from build123d import *

# Parameters (mm, degrees)
F0_W     = 6.858
F0_H     = 2.54
F0_R     = 0.381
F0_W_2   = 0.762
F0_H_2   = 7.62
F1_DEPTH = 2.54


with BuildPart() as f1:
    # F0 (on Top) → F1 (new body)
    with BuildSketch(Plane.XY):
        with Locations((-12.065, 8.001)):
            Rectangle(F0_W, F0_H)
        with Locations((-12.065, -8.001)):
            Rectangle(F0_W, F0_H)
        Polygon((8.636, -13.97), (8.636, 13.97), (-8.636, 13.97), (-8.636, 9.271), (-8.636, 6.731), (-8.636, -6.731), (-8.636, -9.271), (-8.636, -13.97), align=None)
        with Locations((-6.98514, -12.7)):
            Circle(F0_R, mode=Mode.SUBTRACT)
        with Locations((-4.95312, -12.7)):
            Circle(F0_R, mode=Mode.SUBTRACT)
        with Locations((-6.95875, -6.35)):
            Rectangle(F0_W_2, F0_H_2, mode=Mode.SUBTRACT)
        with Locations((-4.9305, -6.35)):
            Rectangle(F0_W_2, F0_H_2, mode=Mode.SUBTRACT)
        with Locations((-2.9211, -12.7)):
            Circle(F0_R, mode=Mode.SUBTRACT)
        with Locations((-0.88908, -12.7)):
            Circle(F0_R, mode=Mode.SUBTRACT)
        with Locations((1.14294, -12.7)):
            Circle(F0_R, mode=Mode.SUBTRACT)
        with Locations((3.17496, -12.7)):
            Circle(F0_R, mode=Mode.SUBTRACT)
        with Locations((5.20698, -12.7)):
            Circle(F0_R, mode=Mode.SUBTRACT)
        with Locations((7.239, -12.7)):
            Circle(F0_R, mode=Mode.SUBTRACT)
        with Locations((-2.90225, -6.35)):
            Rectangle(F0_W_2, F0_H_2, mode=Mode.SUBTRACT)
        with Locations((-0.874, -6.35)):
            Rectangle(F0_W_2, F0_H_2, mode=Mode.SUBTRACT)
        with Locations((1.15425, -6.35)):
            Rectangle(F0_W_2, F0_H_2, mode=Mode.SUBTRACT)
        with Locations((3.1825, -6.35)):
            Rectangle(F0_W_2, F0_H_2, mode=Mode.SUBTRACT)
        with Locations((5.21075, -6.35)):
            Rectangle(F0_W_2, F0_H_2, mode=Mode.SUBTRACT)
        with Locations((7.239, -6.35)):
            Rectangle(F0_W_2, F0_H_2, mode=Mode.SUBTRACT)
        with Locations((-6.95875, 6.35)):
            Rectangle(F0_W_2, F0_H_2, mode=Mode.SUBTRACT)
        with Locations((-4.9305, 6.35)):
            Rectangle(F0_W_2, F0_H_2, mode=Mode.SUBTRACT)
        with Locations((-6.98514, 12.7)):
            Circle(F0_R, mode=Mode.SUBTRACT)
        with Locations((-4.95312, 12.7)):
            Circle(F0_R, mode=Mode.SUBTRACT)
        with Locations((-2.90225, 6.35)):
            Rectangle(F0_W_2, F0_H_2, mode=Mode.SUBTRACT)
        with Locations((-0.874, 6.35)):
            Rectangle(F0_W_2, F0_H_2, mode=Mode.SUBTRACT)
        with Locations((1.15425, 6.35)):
            Rectangle(F0_W_2, F0_H_2, mode=Mode.SUBTRACT)
        with Locations((3.1825, 6.35)):
            Rectangle(F0_W_2, F0_H_2, mode=Mode.SUBTRACT)
        with Locations((5.21075, 6.35)):
            Rectangle(F0_W_2, F0_H_2, mode=Mode.SUBTRACT)
        with Locations((7.239, 6.35)):
            Rectangle(F0_W_2, F0_H_2, mode=Mode.SUBTRACT)
        with Locations((-2.9211, 12.7)):
            Circle(F0_R, mode=Mode.SUBTRACT)
        with Locations((-0.88908, 12.7)):
            Circle(F0_R, mode=Mode.SUBTRACT)
        with Locations((1.14294, 12.7)):
            Circle(F0_R, mode=Mode.SUBTRACT)
        with Locations((3.17496, 12.7)):
            Circle(F0_R, mode=Mode.SUBTRACT)
        with Locations((5.20698, 12.7)):
            Circle(F0_R, mode=Mode.SUBTRACT)
        with Locations((7.239, 12.7)):
            Circle(F0_R, mode=Mode.SUBTRACT)
    extrude(amount=-F1_DEPTH)


solid = f1.part
Work out the finished part from the listing and answer in its coordinate system (mm). A direction names the side the tool comes from. Round coordinates to 2 decimals unless told otherwise and drop trailing zeros. Loops run counter-clockwise (first coordinate to the right, second up) from the corner with the lowest first, then second, coordinate; pieces in that order, holes last. Notation, with made-up numbers: (73.25, 0) -> (127.25, 0) arc R14 cw to (127.25, 16) -> close; hole circle Ø5 at (-5.75, 28). An arc over 180 degrees is marked (long way). Use one line per item in the form item = value.
(1) Straight lines are drawn through the part: line 1 (Y direction, x = -5, z = -0.6); line 2 (Y direction, x = 7, z = -1.15); line 3 (Y direction, x = -13, z = -1). For each, find the intervals that lie inside material, in ascending order.
Answer list:
line_1 = -13.97 to -13.08, -12.32 to -10.16, -2.54 to 2.54, 10.16 to 12.32, 13.08 to 13.97
line_2 = -13.97 to -13, -12.4 to -10.16, -2.54 to 2.54, 10.16 to 12.4, 13 to 13.97
line_3 = -9.27 to -6.73, 6.73 to 9.27
(2) Flat-ended cylindrical pins translate along their axes: P1, Ø1.3, axis at y = 5, z = -0.5, coming from the -X side; P2, Ø3, axis at x = -11, y = 6, coming from the +Z side. Find the tip coordinate at first contact, or state that the pin passes through.
Answer list:
P1 = -8.64
P2 = 0
(3) For a pull along X with two mould halves and no side action, classify faces 5 (the flat face through (-8.636, -12, -1)), 6 (the flat face through (-7.34, 6, -1)), 7 (the flat face through (0, -13.97, -1)), 8 (the flat face through (2.802, -6, -1)) as released by +X, released by -X, zero draft, split by the parting line, or undercut.
Answer list:
face_5 = released by -X
face_6 = undercut
face_7 = zero draft
face_8 = undercut
(4) Find section D-D on y = -12. Give the vertices of the cut face in (x, z).
Answer list:
outline = (-8.64, -2.54) -> (8.64, -2.54) -> (8.64, 0) -> (-8.64, 0) -> close
(5) Find section A-A on x = -11. Give the vertices of the cut face in (y, z).
Answer list:
outline = (-9.27, -2.54) -> (-6.73, -2.54) -> (-6.73, 0) -> (-9.27, 0) -> close; (6.73, -2.54) -> (9.27, -2.54) -> (9.27, 0) -> (6.73, 0) -> close
(6) A tool of negligible diameter and unlimited length cuts with its end or side. For faces 1 (the flat face through (-8.636, 12, -1)), 2 (the flat face through (-12, 6.731, -1)), 3 (the flat face through (-2.521, 6, -1)), 4 (the flat face through (-12, -9.271, -1)), from which of +Z, -Z, +X, -X, +Y, -Y can it reach the whole face along a straight path? Write none if from no direction.
Answer list:
face_1 = +Z, -Z, -X, +Y
face_2 = +Z, -Z, -X
face_3 = +Z, -Z
face_4 = +Z, -Z, -X, -Y
(7) Find section B-B on y = 12.7. Give the number of separate pieces and of enclosed holes in the cut face, then the cut area to 3 significant figures.
Answer list:
separate_pieces = 9
enclosed_holes = 0
area = 28.4 mm2
